Work out the finished part from the listing and answer in its coordinate system (mm). Give positions to 0.01 mm unless a question says otherwise; leave off trailing zeros. Loops run counter-clockwise (first coordinate to the right, second up) from the corner with the lowest first, then second, coordinate; pieces in that order, holes last. Notation, with made-up numbers: (74.5, 83.25) - (94.5, 83.25) arc R22 cw to (94.5, 91.25) - close; hole circle Ø8 at (-16, 55.25). An arc over 180 degrees is marked (long way). Use CSV: the item, a comma, the result in double quotes.
from build123d import *

# Parameters (mm, degrees)
BOSS_EXTRUDE1_DEPTH         = 0.762
F_3_8_0_11_DIAMETER_HOLE1_D = 2.794
FILLET1_R                   = 0.635


with BuildPart() as part:
    # Sketch1 → Boss-Extrude1 (new body)
    with BuildSketch(Plane(origin=(0, 0, 0), x_dir=(1, 0, 0), z_dir=(0, 1, 0))):
        with BuildLine():
            Line((0, 8.128), (-66.294, 8.128))
            ThreePointArc((-66.294, 8.128), (-74.915045876, 4.557045876), (-78.486, -4.064))
            Line((-78.486, -4.064), (-67.056, -4.064))
            ThreePointArc((-67.056, -4.064), (-57.531, -1.524), (-48.006, -4.064))
            Line((-48.006, -4.064), (-39.624, -4.064))
            Line((-39.624, -4.064), (-38.535054482, -8.128))
            Line((-38.535054482, -8.128), (0, -8.128))
            ThreePointArc((0, -8.128), (8.128, 0), (0, 8.128))
        make_face()
    extrude(amount=BOSS_EXTRUDE1_DEPTH)

    # 3/8 (0.11) Diameter Hole1 (through all)
    with Locations(Plane(origin=(0, 0.762, 0), x_dir=(1, 0, 0), z_dir=(0, 1, 0))):
        with Locations((-70.866, 0.254), (-36.503054482, -6.096), (-24.565054482, -3.81), (0, 1.778)):
            Hole(F_3_8_0_11_DIAMETER_HOLE1_D / 2)

    # Fillet1
    fillet1_edges = [part.edges().sort_by_distance(p)[0] for p in [
        (-38.535054482, 0.381, 8.128),
        (-39.624, 0.381, 4.064),
        (-78.486, 0.381, 4.064),
    ]]
    fillet(fillet1_edges, radius=FILLET1_R)


solid = part.part
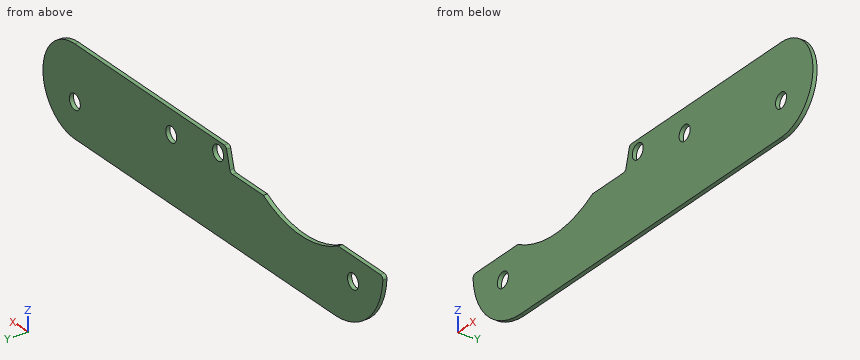
Item 1: A cutting plane is placed at B-B on x = -60.5. Determine the outline of the cut face in (y, z), and give its area (3 significant figures).
Determined:
outline,"(0, -8.13) - (0.76, -8.13) - (0.76, 1.76) - (0, 1.76) - close"
area,"7.53 mm²"
Item 2: A cutting plane is placed at A-A on y = 0.35. Determine the outline of the cut face in (x, z) (3 decimals).
Determined:
outline,"(-78.468, 3.394) arc R12.192 ccw to (-66.294, -8.128) - (0, -8.128) arc R8.128 ccw to (0, 8.128) - (-38.048, 8.128) arc R0.635 ccw to (-38.661, 7.657) - (-39.498, 4.535) arc R0.635 cw to (-40.111, 4.064) - (-48.006, 4.064) arc R19.129 cw to (-67.056, 4.064) - (-77.834, 4.064) arc R0.635 ccw to start; hole circle Ø2.794 at (-70.866, -0.254); hole circle Ø2.794 at (-36.503, 6.096); hole circle Ø2.794 at (-24.565, 3.81); hole circle Ø2.794 at (0, -1.778)"
Item 3: Find the intervals of material crossed by line 1 (X direction, y = 0.2, z = -0.5); line 2 (X direction, y = 0.1, z = -1.5); line 3 (X direction, y = 0.1, z = -2), in increasing order.
Determined:
line 1,"x = -77.6 to -72.24, -69.49 to -0.56, 0.56 to 8.11"
line 2,"x = -77.14 to -71.5, -70.23 to -1.37, 1.37 to 7.99"
line 3,"x = -76.87 to -1.38, 1.38 to 7.88"
Item 4: A cutting plane is placed at C-C on z = -7. Determine the outline of the cut face in (x, y).
Determined:
outline,"(-71.42, 0) - (4.13, 0) - (4.13, 0.76) - (-71.42, 0.76) - close"
